Work out the finished part from the listing and answer in its coordinate system (mm). A direction names the side the tool comes from. Coordinates: 2 decimals unless noted, no trailing zeros. Order: outer loops, then holes, each group sorted by start corner. A loop starts at its lowest first (then second) coordinate and runs counter-clockwise, first axis right, second up. Notation, with made-up numbers: M -14,86.5 L -9,86.5 A36 ccw -9,123.5 Z; hole C -23,59.5 d1. An arc over 180 degrees is marked long. Use a Markdown table: item, result.
from build123d import *

# Parameters (mm, degrees)
BOSS_EXTRUDE1_DEPTH = 2
SKETCH1_4_W         = 58.6
SKETCH1_4_H         = 51.7
BOSS_EXTRUDE2_DEPTH = 20


with BuildPart() as part:
    # Sketch1 → Boss-Extrude1 (new body)
    with BuildSketch(Plane(origin=(0, 0, 0), x_dir=(1, 0, 0), z_dir=(0, 1, 0))):
        Polygon((0, 0), (223.3, 0), (225.3, 0), (225.3, 55.7), (164.7, 55.7), (164.7, 68.2), (46.2, 68.2), (46.2, 81.5), (0, 81.5), align=None)
    extrude(amount=-BOSS_EXTRUDE1_DEPTH)

    # Sketch1<4> → Boss-Extrude2 (add)
    with BuildSketch(Plane(origin=(0, 0, 0), x_dir=(1, 0, 0), z_dir=(0, 1, 0))):
        Polygon((0, 2), (0, 0), (2, 0), (44.2, 0), (46.2, 0), (162.7, 0), (164.7, 0), (223.3, 0), (225.3, 0), (225.3, 2), (225.3, 55.7), (164.7, 55.7), (164.7, 68.2), (46.2, 68.2), (46.2, 81.5), (2, 81.5), (0, 81.5), (0, 79.5), align=None)
        Polygon((162.7, 2), (46.2, 2), (46.2, 66.2), (162.7, 66.2), (162.7, 55.7), (162.7, 53.7), align=None, mode=Mode.SUBTRACT)
        with Locations((194, 27.85)):
            Rectangle(SKETCH1_4_W, SKETCH1_4_H, mode=Mode.SUBTRACT)
        Polygon((2, 2), (2, 79.5), (44.2, 79.5), (44.2, 68.2), (44.2, 66.2), (44.2, 2), align=None, mode=Mode.SUBTRACT)
    extrude(amount=BOSS_EXTRUDE2_DEPTH)


solid = part.part
(1) A cutting plane is placed at B-B (x = 94). Determine the outline of the cut face in (y, z).
Conclusion:
| item | result |
|---|---|
| outline | M -2,-68.2 L 20,-68.2 L 20,-66.2 L 0,-66.2 L 0,-2 L 20,-2 L 20,0 L -2,0 Z |
(2) A cutting plane is placed at D-D (z = -60). Determine the outline of the cut face in (x, y).
Conclusion:
| item | result |
|---|---|
| outline | M 0,-2 L 164.7,-2 L 164.7,20 L 162.7,20 L 162.7,0 L 46.2,0 L 46.2,20 L 44.2,20 L 44.2,0 L 2,0 L 2,20 L 0,20 Z |
(3) A cutting plane is placed at A-A (y = 6.75). Determine the outline of the cut face in (x, z).
Conclusion:
| item | result |
|---|---|
| outline | M 0,-81.5 L 46.2,-81.5 L 46.2,-68.2 L 164.7,-68.2 L 164.7,-55.7 L 225.3,-55.7 L 225.3,0 L 0,0 Z; hole M 2,-79.5 L 44.2,-79.5 L 44.2,-2 L 2,-2 Z; hole M 46.2,-66.2 L 162.7,-66.2 L 162.7,-2 L 46.2,-2 Z; hole M 164.7,-53.7 L 223.3,-53.7 L 223.3,-2 L 164.7,-2 Z |
(4) A cutting plane is placed at C-C (z = -13.5). Determine the outline of the cut face in (x, y).
Conclusion:
| item | result |
|---|---|
| outline | M 0,-2 L 225.3,-2 L 225.3,20 L 223.3,20 L 223.3,0 L 164.7,0 L 164.7,20 L 162.7,20 L 162.7,0 L 46.2,0 L 46.2,20 L 44.2,20 L 44.2,0 L 2,0 L 2,20 L 0,20 Z |
(5) Which of the six approach directions +Z, -Z, +X, -X, +Y, -Y give full straight-line access (tool end or side, diameter ignored) to faces 1 (the flat face through (106, 9, -68.2)), 2 (the flat face through (223.3, 10, -27)), 3 (the flat face through (0, 9, -41))?
Conclusion:
| item | result |
|---|---|
| face 1 | -Z, +X, +Y, -Y |
| face 2 | +Y |
| face 3 | +Z, -Z, -X, +Y, -Y |
(6) Determine the mould class of faces 4 (the flat face through (2, 10, -40)), 5 (the flat face through (23, 9, -81.5)), 6 (the flat face through (194, 10, -53.7)), 7 (the flat face through (225.3, 9, -27)) for opening direction X: pulls with the +X half, pulls with the -X half, needs draft (parallel to the pull), parting line crosses it, or undercut.
Conclusion:
| item | result |
|---|---|
| face 4 | undercut |
| face 5 | needs draft |
| face 6 | undercut |
| face 7 | pulls with the +X half |
(7) Given P1, Ø11, axis at x = 189.5, y = 7.5, coming from the -Z side; P2, Ø10, axis at y = 4.5, z = -61.5, coming from the +X side; P3, Ø1, axis at y = 17.5, z = -72, coming from the +X side, each flat-ended and moving along its own axis, determine where each tip first touches the part or whether it passes through.
Conclusion:
| item | result |
|---|---|
| P1 | z = -55.7 |
| P2 | x = 164.7 |
| P3 | x = 46.2 |
(8) Straight lines are drawn through the part: L1, parallel to X at y = 5.75, z = -7.5; L2, parallel to X at y = 5.75, z = -63.5; L3, parallel to Z at x = 99.5, y = 1.75. For each, find the intervals that lie inside material, in ascending order.
Conclusion:
| item | result |
|---|---|
| L1 | 0 to 2, 44.2 to 46.2, 162.7 to 164.7, 223.3 to 225.3 |
| L2 | 0 to 2, 44.2 to 46.2, 162.7 to 164.7 |
| L3 | -68.2 to -66.2, -2 to 0 |
